Source: CAD feature listing. Evaluate the final solid. Frame: model axes, mm. Give positions to 0.01 mm unless a question says otherwise; leave off trailing zeros. Write each loop counter-clockwise with the first axis right and the second up, starting at its lowest first coordinate (ties: lowest second). Pieces come first, ordered by that corner, then holes. Notation, with made-up numbers: (78.5, -4) - (113.5, -4) arc R23 ccw to (113.5, 23) - close; hole circle Ø1 at (35, -27). An arc over 180 degrees is marked (long way). One line per question, with ' | ' between items. Start each with the question number.
(1) Section C-C, the plane z = 8. Return loops of the section in (x, y).
(2) Ray query, line 1 (X direction, y = 0.5, z = 2.5); line 2 (X direction, y = 1, z = 3); line 3 (Z direction, x = -3, y = 2). Return the intervals inside material, ascending. Write a range as [from, to].
(3) Section A-A, the plane z = 1. Return loops of the section in (x, y), plus the area to 3 significant figures.
(4) Section B-B, the plane y = -1. Return loops of the section in (x, z).
```python
from build123d import *
from build123d.topology import SkipClean

# Parameters (mm, degrees)
SKETCH_2_W      = 60.888503838
SKETCH_2_H      = 32.359912294
EXTRUDE_1_DEPTH = 10


with BuildPart() as part:
    # 草图2 → 凸台-拉伸1 (new body)
    with BuildSketch(Plane.XY):
        Rectangle(SKETCH_2_W, SKETCH_2_H)
    extrude(amount=EXTRUDE_1_DEPTH)

    # 草图5 → 切除-旋转5 (revolve, cut)
    with BuildSketch(Plane(origin=(0, 0, 0), x_dir=(1, 0, 0), z_dir=(0, 1, 0))):
        with BuildLine():
            Line((-30.444251919, 0), (-30.444251919, -10))
            ThreePointArc((-30.444251919, -10), (-25.444251919, -5), (-30.444251919, 0))
        make_face()
    cut_revolve_5 = revolve(axis=Axis((-30.444251919, 0, 0), (0, 0, 1)), mode=Mode.SUBTRACT)

    # 镜向1: 切除-旋转5 across plane
    with SkipClean():  # the faces are left unmerged after this step: merging them gives an invalid solid
        add(cut_revolve_5.mirror(Plane(origin=(0, 0, 0), x_dir=(0, 0, 1), z_dir=(1, 0, 0))), mode=Mode.SUBTRACT)

    # 草图6 → 切除-旋转6 (revolve, cut)
    with SkipClean():  # the faces are left unmerged after this step: merging them gives an invalid solid
        with BuildSketch(Plane(origin=(0, 0, 0), x_dir=(1, 0, 0), z_dir=(0, 1, 0))):
            with BuildLine():
                Line((-4.913926023, 0), (4.913926023, 0))
                ThreePointArc((4.913926023, 0), (0, -4.913926023), (-4.913926023, 0))
            make_face()
        revolve(axis=Axis((-4.913926023, 0, 0), (1, 0, 0)), mode=Mode.SUBTRACT)


solid = part.part
```
Check sheet entries:
1) outline: (-30.44, -16.18) - (30.44, -16.18) - (30.44, -4) arc R4 cw to (30.44, 4) - (30.44, 16.18) - (-30.44, 16.18) - (-30.44, 4) arc R4 cw to (-30.44, -4) - close
2) line 1: [-26.14, -4.2], [4.2, 26.14] | line 2: [-25.97, -3.76], [3.76, 25.97] | line 3: [3.34, 10]
3) outline: (-30.44, -16.18) - (30.44, -16.18) - (30.44, -3) arc R3 cw to (30.44, 3) - (30.44, 16.18) - (-30.44, 16.18) - (-30.44, 3) arc R3 cw to (-30.44, -3) - close; hole circle Ø9.62 at (0, 0) | area: 1,870 mm²
4) outline: (-30.44, 0) - (-4.81, 0) arc R4.81 cw to (4.81, 0) - (30.44, 0) - (30.44, 0.1) arc R4.9 cw to (30.44, 9.9) - (30.44, 10) - (-30.44, 10) - (-30.44, 9.9) arc R4.9 cw to (-30.44, 0.1) - close
